Part print with two shaded views. Sizes in mm from the minimum x, y, z corner. Round coordinates to 2 decimals unless told otherwise and drop trailing zeros. Write each loop counter-clockwise with the first axis right and the second up, starting at its lowest first coordinate (ties: lowest second). Pieces come first, ordered by that corner, then holes. Notation, with made-up numbers: (-15, -17.5) -> (-9, -17.5) arc R11 ccw to (-9, -8.5) -> close; hole circle Ø10 at (25, -35.75). An arc over 180 degrees is marked (long way). Answer as CSV lines item,"result".
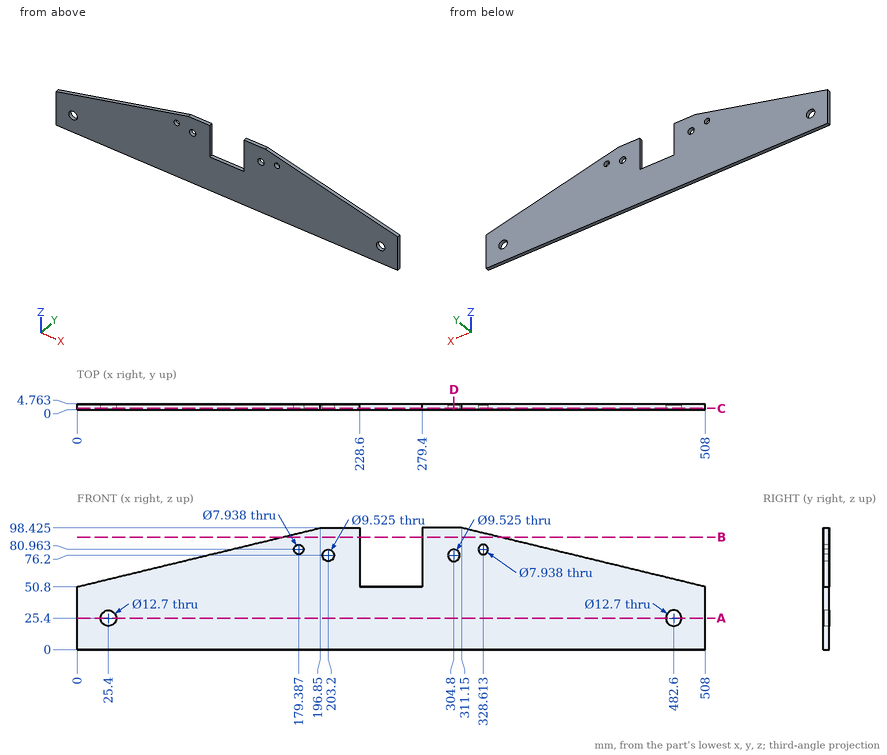
1. Cut at D-D, the plane x = 304.8. Write the cut outline in (y, z) (1 decimal).
Results found:
outline,"(0, 0) -> (4.8, 0) -> (4.8, 71.4) -> (0, 71.4) -> close; (0, 81) -> (4.8, 81) -> (4.8, 98.4) -> (0, 98.4) -> close"
2. Probe line 1 along Z through (x, y) = (203.2, 3.05) (1 decimal); line 2 along Z through (x, y) = (85.5, 0.2) (1 decimal); line 3 along Z through (x, y) = (201, 0.4) (1 decimal). List the from-to ranges inside material, lowest first.
Results found:
line 1,"z = 0 to 71.4, 81 to 98.4"
line 2,"z = 0 to 71.5"
line 3,"z = 0 to 72, 80.4 to 98.4"
3. Cut at C-C, the plane y = 1.25. Count the separate pieces of the cut face and the enclosed holes in it, then the cut area to 3 significant figures.
Results found:
separate pieces,"1"
enclosed holes,"6"
area,"37,700 mm2"
4. Drop flat-ended pins along their axis: pin 1 Ø1.4 at (x, y) = (250, 3) entering from +Z; pin 2 Ø12.5 at (x, z) = (203.2, 76.2) entering from +Y; pin 3 Ø5 at (x, z) = (179.39, 80.96) entering from -Y; pin 4 Ø1 at (x, y) = (65, 4) entering from +Z. Give the stop position or say it passes through.
Results found:
pin 1,"stops at z = 50.8"
pin 2,"stops at y = 4.76"
pin 3,"passes through"
pin 4,"stops at z = 66.65"
5. Cut at A-A, the plane z = 25.4. Write the cut outline in (x, y).
Results found:
outline,"(0, 0) -> (19.05, 0) -> (19.05, 4.76) -> (0, 4.76) -> close; (31.75, 0) -> (476.25, 0) -> (476.25, 4.76) -> (31.75, 4.76) -> close; (488.95, 0) -> (508, 0) -> (508, 4.76) -> (488.95, 4.76) -> close"
6. Cut at B-B, the plane z = 91. Write the cut outline in (x, y).
Results found:
outline,"(166.16, 0) -> (228.6, 0) -> (228.6, 4.76) -> (166.16, 4.76) -> close; (279.4, 0) -> (341.84, 0) -> (341.84, 4.76) -> (279.4, 4.76) -> close"
